Read the model definition and answer for the solid it produces. Units are mm, in the model's axes. A direction names the side the tool comes from. Round coordinates to 2 decimals unless told otherwise and drop trailing zeros. Order: outer loops, then holes, each group sorted by start corner. A loop starts at its lowest first (then second) coordinate and runs counter-clockwise, first axis right, second up. Notation, with made-up numbers: (77, -15) -> (90, -15) arc R11 cw to (90, -9) -> close; hole circle Ø10 at (78, 14). An arc over 180 degrees is marked (long way). One line per item, written item: value. Start each with the question number.
1. Section A-A (y = 4.75) is taken. Give the vertices of the cut face in (x, z).
2. For faces 1 (the face through (-129.99, 4.93, -130.15)), 2 (the face through (153, 10, -2)), determine the directions among +Z, -Z, +X, -X, +Y, -Y from which every point of the face is accessible in a straight line to the end or side of a thin tool.
3. Consider line 1 (X direction, y = 2.25, z = 21.5); line 2 (X direction, y = 8.5, z = 126). Determine where each line is inside the solid, lowest interval first.
4. Section B-B (z = 76.5) is taken. Give the vertices of the cut face in (x, y), then the cut area to 3 significant figures.
5. The mould has two halves that part along Z. Classify faces 3 (the face through (-129.99, 4.93, 130.15)), 4 (the face through (153, 0, -2)), 5 (the face through (130.15, 4.93, -129.99)), 6 (the face through (-172.15, 5.07, 171.99)): released by +Z, released by -Z, zero draft, split by the parting line, or undercut.
6. Section C-C (x = 24) is taken. Give the vertices of the cut face in (y, z), then the cut area to 3 significant figures.
from build123d import *

# Parameters (mm, degrees)
SKETCH1_W           = 350
SKETCH1_H           = 350
BOSS_EXTRUDE1_DEPTH = 10
SKETCH2_W           = 266
SKETCH2_H           = 266
CUT_EXTRUDE1_DEPTH  = 248.68932153
FILLET1_R           = 10


with BuildPart() as part:
    # Sketch1 → Boss-Extrude1 (new body)
    with BuildSketch(Plane(origin=(0, 0, 0), x_dir=(1, 0, 0), z_dir=(0, 1, 0))):
        Rectangle(SKETCH1_W, SKETCH1_H)
    extrude(amount=BOSS_EXTRUDE1_DEPTH)

    # Sketch2 → Cut-Extrude1 (cut, through all)
    with BuildSketch(Plane(origin=(0, 10, 0), x_dir=(1, 0, 0), z_dir=(0, 1, 0))):
        Rectangle(SKETCH2_W, SKETCH2_H)
    extrude(amount=-CUT_EXTRUDE1_DEPTH, mode=Mode.SUBTRACT)

    # Fillet1
    fillet1_edges = [part.edges().sort_by_distance(p)[0] for p in [
        (133, 5, -133),
        (133, 5, 133),
        (-133, 5, 133),
        (-133, 5, -133),
        (175, 5, 175),
        (-175, 5, 175),
        (-175, 5, -175),
        (175, 5, -175),
    ]]
    fillet(fillet1_edges, radius=FILLET1_R)


solid = part.part
Answer:
1. outline: (-175, -165) arc R10 ccw to (-165, -175) -> (165, -175) arc R10 ccw to (175, -165) -> (175, 165) arc R10 ccw to (165, 175) -> (-165, 175) arc R10 ccw to (-175, 165) -> close; hole (-133, -123) arc R10 ccw to (-123, -133) -> (123, -133) arc R10 ccw to (133, -123) -> (133, 123) arc R10 ccw to (123, 133) -> (-123, 133) arc R10 ccw to (-133, 123) -> close
2. face 1: +Y, -Y
2. face 2: +Z, -Z, +X, -X, +Y
3. line 1: -175 to -133, 133 to 175
3. line 2: -175 to -132.54, 132.54 to 175
4. outline: (-175, 0) -> (-133, 0) -> (-133, 10) -> (-175, 10) -> close; (133, 0) -> (175, 0) -> (175, 10) -> (133, 10) -> close
4. area: 840 mm^2
5. face 3: undercut
5. face 4: zero draft
5. face 5: undercut
5. face 6: released by +Z
6. outline: (0, -175) -> (10, -175) -> (10, -133) -> (0, -133) -> close; (0, 133) -> (10, 133) -> (10, 175) -> (0, 175) -> close
6. area: 840 mm^2
